Work out the finished part from the listing and answer in its coordinate system (mm). A direction names the side the tool comes from. Coordinates: 2 decimals unless noted, no trailing zeros. Answer as CSV lines item,"result". Start each with the question number.
Item 1: Straight lines are drawn through the part: L1, parallel to Y at x = 41.5, z = 34; L2, parallel to Y at x = -67.5, z = 19.5; L3, parallel to X at y = -73.5, z = 18.5. For each, find the intervals that lie inside material, in ascending order.
Item 2: Which of the six approach directions +Z, -Z, +X, -X, +Y, -Y give full straight-line access (tool end or side, diameter ignored) to faces 4 (the face through (96.49, 96.85, 20.28)), 5 (the face through (106.04, 105.47, 20.28))?
Item 3: For a pull along X with two mould halves and no side action, classify faces 1 (the face through (-106.04, -105.47, 20.28)), 2 (the face through (-96.49, -96.85, 20.28)), 3 (the face through (1, -109, 40)) as pulls with the +X half, pulls with the -X half, needs draft (parallel to the pull), parting line crosses it, or undercut.
Item 4: Each of these flat-tipped pins is pushed along its axis until it touches: pin 1 Ø4 at (y, z) = (-55, 24.5) entering from -X; pin 2 Ø3 at (y, z) = (49.5, 11) entering from +X; pin 3 Ø6 at (y, z) = (-8, 27.5) entering from +X. Where does it stop, or does it pass through?
```python
from build123d import *

# Parameters (mm, degrees)
F1_DEPTH = 40
F1_TAPER = 10


with BuildPart() as f1:
    # F0 (on Top) → F1 (new body)
    with BuildSketch(Plane.XY):
        with BuildLine():
            Line((80, 120), (-120, 120))
            Line((-120, 120), (-120, -80))
            ThreePointArc((-120, -80), (-108.2842712475, -108.2842712475), (-80, -120))
            Line((-80, -120), (120, -120))
            Line((120, -120), (120, 80))
            ThreePointArc((120, 80), (108.2842712475, 108.2842712475), (80, 120))
        make_face()
        with BuildLine():
            Line((-100, 100), (80, 100))
            ThreePointArc((80, 100), (94.1421356237, 94.1421356237), (100, 80))
            Line((100, 80), (100, -100))
            Line((100, -100), (-80, -100))
            ThreePointArc((-80, -100), (-94.1421356237, -94.1421356237), (-100, -80))
            Line((-100, -80), (-100, 100))
        make_face(mode=Mode.SUBTRACT)
    extrude(amount=F1_DEPTH, taper=F1_TAPER)


solid = f1.part
```
Checked values:
1,L1,"y = -114 to -106, 106 to 114"
1,L2,"y = -116.56 to -103.44, 103.44 to 116.56"
1,L3,"x = -116.74 to -103.26, 103.26 to 116.74"
2,face 4,"+Z"
2,face 5,"+Z, +X, +Y"
3,face 1,"pulls with the -X half"
3,face 2,"undercut"
3,face 3,"needs draft"
4,pin 1,"stops at x = -116.03"
4,pin 2,"stops at x = 118.32"
4,pin 3,"stops at x = 115.68"
